```python
from build123d import *

# Parameters (mm, degrees)
CYLINDER028_R           = 1.5
CYLINDER028_DEPTH       = 10
CYLINDER028_PITCH_ANGLE = 90
CYLINDER023_R           = 2.4
CYLINDER023_DEPTH       = 3
CYLINDER026_R           = 0.9
CYLINDER026_DEPTH       = 3
CYLINDER027_R           = 0.9
CYLINDER027_DEPTH       = 3
CYLINDER025_R           = 2.4
CYLINDER025_DEPTH       = 6
CYLINDER024_R           = 2.4
CYLINDER024_DEPTH       = 5
BOX042_W                = 2
BOX042_H                = 32
BOX042_DEPTH            = 10
BOX041_W                = 6
BOX041_H                = 9
BOX041_DEPTH            = 10
BOX040_W                = 6
BOX040_H                = 9
BOX040_DEPTH            = 10
BOX039_W                = 24.5
BOX039_H                = 40
BOX039_DEPTH            = 2


with BuildPart() as cilindro028:
    # Cylinder028 → Cylinder028 (new body)
    with BuildSketch(Plane.XY):
        Circle(CYLINDER028_R)
    extrude(amount=CYLINDER028_DEPTH)


with BuildPart() as cilindro028_1:
    # Cylinder028 pitch: moved
    add(cilindro028.part.rotate(Axis((0, 0, 0), (0, 1, 0)), CYLINDER028_PITCH_ANGLE))


with BuildPart() as cilindro028_2:
    # Cylinder028 placement: moved
    add(cilindro028_1.part.moved(Location((-49, -0.5, 6))))


with BuildPart() as cilindro023:
    # Cylinder023 → Cylinder023 (new body)
    with BuildSketch(Plane(origin=(-59.5, -0.5, 0), x_dir=(1, 0, 0), z_dir=(0, 0, 1))):
        Circle(CYLINDER023_R)
    extrude(amount=CYLINDER023_DEPTH)


with BuildPart() as cilindro026:
    # Cylinder026 → Cylinder026 (new body)
    with BuildSketch(Plane(origin=(-49.5, 9.5, 0), x_dir=(1, 0, 0), z_dir=(0, 0, 1))):
        Circle(CYLINDER026_R)
    extrude(amount=CYLINDER026_DEPTH)


with BuildPart() as cilindro027:
    # Cylinder027 → Cylinder027 (new body)
    with BuildSketch(Plane(origin=(-49.5, -10.5, 0), x_dir=(1, 0, 0), z_dir=(0, 0, 1))):
        Circle(CYLINDER027_R)
    extrude(amount=CYLINDER027_DEPTH)


with BuildPart() as cilindro025:
    # Cylinder025 → Cylinder025 (new body)
    with BuildSketch(Plane(origin=(-59.5, -20.5, -4), x_dir=(1, 0, 0), z_dir=(0, 0, 1))):
        Circle(CYLINDER025_R)
    extrude(amount=CYLINDER025_DEPTH)


with BuildPart() as cilindro024:
    # Cylinder024 → Cylinder024 (new body)
    with BuildSketch(Plane(origin=(-59.5, 19.5, -3), x_dir=(1, 0, 0), z_dir=(0, 0, 1))):
        Circle(CYLINDER024_R)
    extrude(amount=CYLINDER024_DEPTH)


with BuildPart() as cubo036:
    # Box042 → Box042 (new body)
    with BuildSketch(Plane(origin=(-47, -17, 0), x_dir=(1, 0, 0), z_dir=(0, 0, 1))):
        with Locations((1, 16)):
            Rectangle(BOX042_W, BOX042_H)
    extrude(amount=BOX042_DEPTH)


with BuildPart() as cubo035:
    # Box041 → Box041 (new body)
    with BuildSketch(Plane(origin=(-68, 5, -3), x_dir=(1, 0, 0), z_dir=(0, 0, 1))):
        with Locations((3, 4.5)):
            Rectangle(BOX041_W, BOX041_H)
    extrude(amount=BOX041_DEPTH)


with BuildPart() as cubo034:
    # Box040 → Box040 (new body)
    with BuildSketch(Plane(origin=(-68, -15, -3), x_dir=(1, 0, 0), z_dir=(0, 0, 1))):
        with Locations((3, 4.5)):
            Rectangle(BOX040_W, BOX040_H)
    extrude(amount=BOX040_DEPTH)


with BuildPart() as obj1:
    # Box039 → Box039 (new body)
    with BuildSketch(Plane(origin=(-69.5, -20.5, -2), x_dir=(1, 0, 0), z_dir=(0, 0, 1))):
        with Locations((12.25, 20)):
            Rectangle(BOX039_W, BOX039_H)
    extrude(amount=BOX039_DEPTH)

    # Cut049: cut Cubo034
    add(cubo034.part, mode=Mode.SUBTRACT)

    # Cut050: cut Cubo035
    add(cubo035.part, mode=Mode.SUBTRACT)

    # Fusion011: union Cubo036
    add(cubo036.part)

    # Cut051: cut Cilindro024
    add(cilindro024.part, mode=Mode.SUBTRACT)

    # Cut052: cut Cilindro025
    add(cilindro025.part, mode=Mode.SUBTRACT)

    # Fusion012: union Cilindro023, Cilindro026, Cilindro027
    add(cilindro023.part)
    add(cilindro026.part)
    add(cilindro027.part)

    # Cut053: cut Cilindro028
    add(cilindro028_2.part, mode=Mode.SUBTRACT)


solid = obj1.part
```
Part model, mm, in its own coordinate system. A direction names the side the tool comes from. Round coordinates to 2 decimals unless told otherwise and drop trailing zeros. Loops run counter-clockwise (first coordinate to the right, second up) from the corner with the lowest first, then second, coordinate; pieces in that order, holes last.
Item 1: Drop flat-ended pins along their axis: P1, Ø0.6, axis at x = -45.5, z = 7, coming from the +Y side; P2, Ø2, axis at x = -49.5, y = -11, coming from the +Z side; P3, Ø4, axis at y = -0.5, z = 6, coming from the -X side; P4, Ø2, axis at x = -64.5, y = -8, coming from the +Z side. Give the stop position or say it passes through.
Item 2: 3-axis set-ups, long thin cutter, end or side, ignore diameter. For faces 1 (the face through (-68, 9, -1)), 2 (the face through (-60, 0, 3)), 3 (the face through (-50.4, 9.5, 1.5)): which of +Z, -Z, +X, -X, +Y, -Y reach the whole face in a straight line?
Item 3: Mould opens along X. For faces 4 (the face through (-66, -20.5, -1)), 5 (the face through (-45, -1, 4)), 6 (the face through (-57.283, -1.419, 1.479)) say: +X half, -X half, draft (parallel to the pull), parting line (faces both ways), or undercut.
Item 4: Cut at C-C, the plane y = -12. Give the cut face in (x, z), then the cut area to 3 significant figures.
Item 5: Cut at B-B, the plane z = 6. Give the cut face in (x, y).
Item 6: Drill centre lines: line 1 (X direction, y = 9, z = -1.5); line 2 (Y direction, x = -46.2, z = 6); line 3 (Z direction, x = -45.85, y = -0.5). Where is each one in solid material? Low to high.
Item 7: Cut at D-D, the plane z = 2.5. Give the cut face in (x, y), then the cut area to 3 significant figures.
Item 8: Cut at A-A, the plane x = -64.75. Give the cut face in (y, z), then the cut area to 3 significant figures.
A:
1. P1: stops at y = 15
1. P2: stops at z = 3
1. P3: stops at x = -47
1. P4: passes through
2. face 1: +Z, -Z
2. face 2: +Z, -X, +Y, -Y
2. face 3: +Z
3. face 4: draft
3. face 5: +X half
3. face 6: undercut
4. outline: (-69.5, -2) - (-68, -2) - (-68, 0) - (-69.5, 0) - close; (-62, -2) - (-45, -2) - (-45, 10) - (-47, 10) - (-47, 0) - (-62, 0) - close
4. area: 57.0 mm2
5. outline: (-47, -17) - (-45, -17) - (-45, -2) - (-47, -2) - close; (-47, 1) - (-45, 1) - (-45, 15) - (-47, 15) - close
6. line 1: x = -69.5 to -68, -62 to -45
6. line 2: y = -17 to -2, 1 to 15
6. line 3: z = -2 to 4.5, 7.5 to 10
7. outline: circle Ø4.8 at (-59.5, -0.5); circle Ø1.8 at (-49.5, -10.5); circle Ø1.8 at (-49.5, 9.5); (-47, -17) - (-45, -17) - (-45, 15) - (-47, 15) - close
7. area: 87.2 mm2
8. outline: (-20.5, -2) - (-15, -2) - (-15, 0) - (-20.5, 0) - close; (-6, -2) - (5, -2) - (5, 0) - (-6, 0) - close; (14, -2) - (19.5, -2) - (19.5, 0) - (14, 0) - close
8. area: 44.0 mm2
